from build123d import *

# Parameters (mm, degrees)
SKETCH1_W           = 247.65
SKETCH1_H           = 88.9
BOSS_EXTRUDE1_DEPTH = 171.45
SHELL1_T            = -2.54
BOSS_EXTRUDE2_DEPTH = 101.6
CUT_EXTRUDE1_REACH  = 23.59
SKETCH4_R           = 25.4
SKETCH5_W           = 6.35
SKETCH5_H           = 64.77
SKETCH5_H_2         = 83.82
BOSS_EXTRUDE3_DEPTH = 101.6


with BuildPart() as part:
    # Sketch1 → Boss-Extrude1 (new body)
    with BuildSketch(Plane(origin=(0, 0, 0), x_dir=(1, 0, 0), z_dir=(0, 1, 0))):
        with Locations((123.825, -44.45)):
            Rectangle(SKETCH1_W, SKETCH1_H)
    extrude(amount=BOSS_EXTRUDE1_DEPTH)

    # Shell1
    shell1_openings = [part.faces().sort_by_distance(p)[0] for p in [
        (123.825, 171.45, 44.45),
    ]]
    offset(amount=SHELL1_T, openings=shell1_openings, kind=Kind.INTERSECTION)

    # Sketch2 → Boss-Extrude2 (add)
    with BuildSketch(Plane(origin=(0, 2.54, 0), x_dir=(1, 0, 0), z_dir=(0, 1, 0))):
        Polygon((245.11, -73.66), (156.21, -73.66), (156.21, -86.36), (149.86, -86.36), (149.86, -67.31), (245.11, -67.31), align=None)
    extrude(amount=BOSS_EXTRUDE2_DEPTH)

    # Sketch4 → Cut-Extrude1 (cut, up to next)
    with BuildSketch(Plane(origin=(0, 0, 67.31), x_dir=(-1, 0, 0), z_dir=(0, 0, -1)), mode=Mode.PRIVATE) as cut_extrude1_sk1:
        with Locations((-197.485, 104.14)):
            Circle(SKETCH4_R)
    cut_extrude1_tool1 = extrude(cut_extrude1_sk1.sketch, amount=-CUT_EXTRUDE1_REACH, mode=Mode.PRIVATE) & part.part
    add(cut_extrude1_tool1.solids().sort_by_distance((197.485, 104.14, 67.31))[0], mode=Mode.SUBTRACT)

    # Sketch5 → Boss-Extrude3 (add)
    with BuildSketch(Plane(origin=(0, 2.54, 0), x_dir=(1, 0, 0), z_dir=(0, 1, 0))):
        with Locations((153.035, -34.925)):
            Rectangle(SKETCH5_W, SKETCH5_H)
        with Locations((69.215, -44.45)):
            Rectangle(SKETCH5_W, SKETCH5_H_2)
    extrude(amount=BOSS_EXTRUDE3_DEPTH)


solid = part.part
Input: part model. Units: mm. Frame: model coordinates. A direction names the side the tool comes from. Coordinates: 2 decimals unless noted, no trailing zeros. Write each loop counter-clockwise with the first axis right and the second up, starting at its lowest first coordinate (ties: lowest second). Pieces come first, ordered by that corner, then holes. Notation, with made-up numbers: M 8.25,28.5 L 44.25,28.5 A22 cw 44.25,63.5 Z; hole C 30.25,68 d7. An arc over 180 degrees is marked long. Answer as a JSON object with one key per item and string values. Group by question number.
(1) Section A-A on y = 120. Output: boundary loops of the cut face in (x, z).
(2) Ray query, line 1 along X through (y, z) = (50, 71); line 2 along X through (y, z) = (55, 43.5); line 3 along Z through (x, y) = (16.5, 155). Return the intervals inside material, ascending. Write a range as [from, to].
(3) Set-up query: faces 1 (the face through (66.04, 53, 45)), 2 (the face through (122, 85, 0)). Return all of +Z, -Z, +X, -X, +Y, -Y with unobstructed straight access to the full face (end or side cutting, diameter ignored); none if empty.
(4) Section D-D on y = 40.5. Output: boundary loops of the cut face in (x, z), plus the area to 3 significant figures.
(5) Mould query, pull axis X, two halves, no side actions, for faces 3 (the face through (72.39, 53, 45)), 4 (the face through (201, 53, 73.66)), 5 (the face through (122, 0, 44)). Classes: pulls with the +X half, pulls with the -X half, needs draft (parallel to the pull), parting line crosses it, or undercut.
(6) Section B-B on z = 25. Output: boundary loops of the cut face in (x, y).
(7) Contact query for flat-ended pins moving along their axis: P1, Ø10, axis at x = 83, y = 73, coming from the -Z side; P2, Ø1.5, axis at x = 102.5, z = 70, coming from the +Y side; P3, Ø3, axis at x = 69, z = 55.5, coming from the +Y side. Output: stop coordinate, or through.
(8) Section C-C on x = 142.5. Output: boundary loops of the cut face in (y, z), plus the area to 3 significant figures.
Result set:
{
 "1": {"outline": "M 0,0 L 247.65,0 L 247.65,88.9 L 0,88.9 Z; hole M 2.54,2.54 L 245.11,2.54 L 245.11,86.36 L 2.54,86.36 Z"},
 "2": {"line 1": "x = [0, 2.54], [66.04, 72.39], [149.86, 247.65]", "line 2": "x = [0, 2.54], [66.04, 72.39], [149.86, 156.21], [245.11, 247.65]", "line 3": "z = [0, 2.54], [86.36, 88.9]"},
 "3": {"face 1": "+Y", "face 2": "-Z, +X, -X, +Y, -Y"},
 "4": {"outline": "M 0,0 L 247.65,0 L 247.65,88.9 L 0,88.9 Z; hole M 2.54,2.54 L 66.04,2.54 L 66.04,86.36 L 2.54,86.36 Z; hole M 72.39,2.54 L 149.86,2.54 L 149.86,86.36 L 72.39,86.36 Z; hole M 156.21,2.54 L 245.11,2.54 L 245.11,67.31 L 156.21,67.31 Z; hole M 156.21,73.66 L 245.11,73.66 L 245.11,86.36 L 156.21,86.36 Z", "area": "3,310 mm2"},
 "5": {"face 3": "undercut", "face 4": "undercut", "face 5": "needs draft"},
 "6": {"outline": "M 0,0 L 247.65,0 L 247.65,171.45 L 245.11,171.45 L 245.11,2.54 L 156.21,2.54 L 156.21,104.14 L 149.86,104.14 L 149.86,2.54 L 72.39,2.54 L 72.39,104.14 L 66.04,104.14 L 66.04,2.54 L 2.54,2.54 L 2.54,171.45 L 0,171.45 Z"},
 "7": {"P1": "stops at z = 0", "P2": "stops at y = 2.54", "P3": "stops at y = 104.14"},
 "8": {"outline": "M 0,0 L 171.45,0 L 171.45,2.54 L 2.54,2.54 L 2.54,86.36 L 171.45,86.36 L 171.45,88.9 L 0,88.9 Z", "area": "1,080 mm2"}
}
